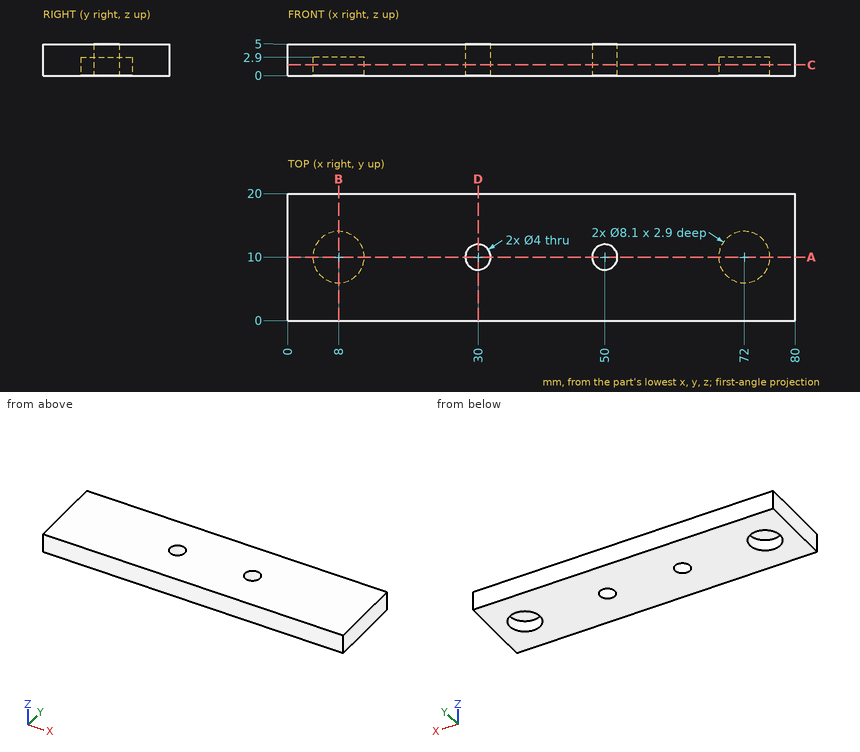
Drawing for the job (mm, zero at the part's lowest x, y, z). Round coordinates to 2 decimals unless told otherwise and drop trailing zeros. Loops run counter-clockwise (first coordinate to the right, second up) from the corner with the lowest first, then second, coordinate; pieces in that order, holes last. Notation, with made-up numbers: (-3, 74.25) -> (9, 74.25) arc R18 ccw to (9, 88.25) -> close; hole circle Ø4 at (47.5, -9). An arc over 180 degrees is marked (long way). Use one line per item in the form item = value. Start each with the question number.
Item 1: Band-saw the part on B-B (x = 8). List the corners of the cut face in (y, z), plus the area to 3 significant figures.
Item 2: Drop a flat-ended pin along its axis: pin 1 Ø2.5 at (x, y) = (71.5, 12) entering from -Z. Give the stop position or say it passes through.
Item 3: Drill centre lines: line 1 along Y through (x, z) = (30, 1.7); line 2 along X through (y, z) = (10.5, 1.75); line 3 along Y through (x, z) = (72, 0.95). Where is each one in solid material? Low to high.
Item 4: Band-saw the part on D-D (x = 30). List the corners of the cut face in (y, z).
Item 5: Band-saw the part on C-C (z = 1.7). List the corners of the cut face in (x, y), plus the area to 3 significant figures.
Item 6: Band-saw the part on A-A (y = 10). List the corners of the cut face in (x, z), plus the area to 3 significant figures.
Data:
q1.outline = (0, 0) -> (5.95, 0) -> (5.95, 2.9) -> (14.05, 2.9) -> (14.05, 0) -> (20, 0) -> (20, 5) -> (0, 5) -> close
q1.area = 76.5 mm^2
q2.pin_1 = 2.9
q3.line_1 = 0 to 8, 12 to 20
q3.line_2 = 0 to 3.98, 12.02 to 28.06, 31.94 to 48.06, 51.94 to 67.98, 76.02 to 80
q3.line_3 = 0 to 5.95, 14.05 to 20
q4.outline = (0, 0) -> (8, 0) -> (8, 5) -> (0, 5) -> close; (12, 0) -> (20, 0) -> (20, 5) -> (12, 5) -> close
q5.outline = (0, 0) -> (80, 0) -> (80, 20) -> (0, 20) -> close; hole circle Ø8.1 at (8, 10); hole circle Ø4 at (30, 10); hole circle Ø4 at (50, 10); hole circle Ø8.1 at (72, 10)
q5.area = 1,470 mm^2
q6.outline = (0, 0) -> (3.95, 0) -> (3.95, 2.9) -> (12.05, 2.9) -> (12.05, 0) -> (28, 0) -> (28, 5) -> (0, 5) -> close; (32, 0) -> (48, 0) -> (48, 5) -> (32, 5) -> close; (52, 0) -> (67.95, 0) -> (67.95, 2.9) -> (76.05, 2.9) -> (76.05, 0) -> (80, 0) -> (80, 5) -> (52, 5) -> close
q6.area = 313 mm^2
